The figure shows three views and two pictorial views of one solid part (mm, origin at its lowest corner). Answer the questions. Give positions to 0.01 mm unless a question says otherwise; leave off trailing zeros. Loops run counter-clockwise (first coordinate to the right, second up) from the corner with the lowest first, then second, coordinate; pieces in that order, holes last. Notation, with made-up numbers: (23, -14.75) - (82, -14.75) arc R7 ccw to (82, -9.75) - close; hole circle Ø2 at (34.5, 17.5). An arc over 180 degrees is marked (long way). Write item = value, one per line.
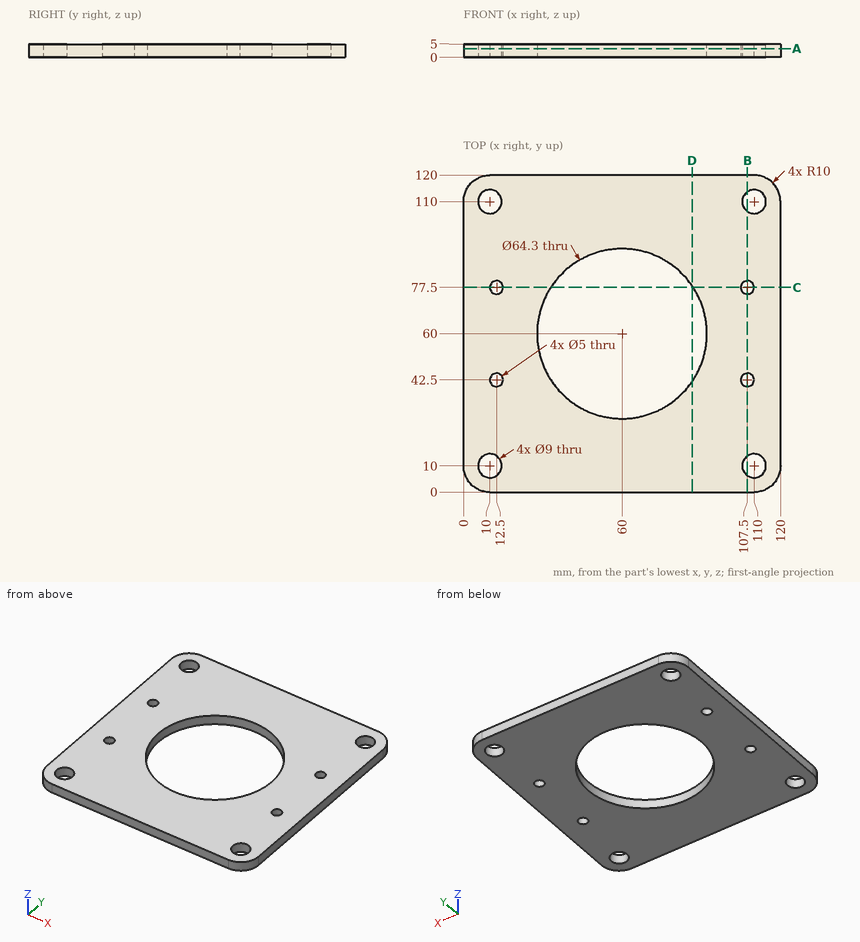
1) Find the intervals of material crossed by probe 1 along X at (y, z) = (6.5, 0.8); probe 2 along Y at (x, z) = (106, 4.4); probe 3 along Y at (x, z) = (74, 0.6), in increasing order.
Output:
probe_1 = 0.63 to 7.17, 12.83 to 107.17, 112.83 to 119.37
probe_2 = 0 to 7.94, 12.06 to 40.5, 44.5 to 75.5, 79.5 to 107.94, 112.06 to 120
probe_3 = 0 to 31.06, 88.94 to 120
2) A cutting plane is placed at C-C on y = 77.5. Determine the outline of the cut face in (x, z), then the cut area to 3 significant figures.
Output:
outline = (0, 0) - (10, 0) - (10, 5) - (0, 5) - close; (15, 0) - (33.03, 0) - (33.03, 5) - (15, 5) - close; (86.97, 0) - (105, 0) - (105, 5) - (86.97, 5) - close; (110, 0) - (120, 0) - (120, 5) - (110, 5) - close
area = 280 mm²
3) A cutting plane is placed at B-B on x = 107.5. Determine the outline of the cut face in (y, z), then the cut area to 3 significant figures.
Output:
outline = (0, 0) - (6.26, 0) - (6.26, 5) - (0, 5) - close; (13.74, 0) - (40, 0) - (40, 5) - (13.74, 5) - close; (45, 0) - (75, 0) - (75, 5) - (45, 5) - close; (80, 0) - (106.26, 0) - (106.26, 5) - (80, 5) - close; (113.74, 0) - (120, 0) - (120, 5) - (113.74, 5) - close
area = 475 mm²
4) A cutting plane is placed at A-A on z = 3.25. Give the number of separate pieces and of enclosed holes in the cut face, then the cut area to 3 significant figures.
Output:
separate_pieces = 1
enclosed_holes = 9
area = 10,700 mm²
5) A cutting plane is placed at D-D on x = 86.5. Determine the outline of the cut face in (y, z), then the cut area to 3 significant figures.
Output:
outline = (0, 0) - (41.8, 0) - (41.8, 5) - (0, 5) - close; (78.2, 0) - (120, 0) - (120, 5) - (78.2, 5) - close
area = 418 mm²
6) This flat-tipped pin is pushed along its axis until it touches: P1, Ø8, axis at x = 10, y = 110, coming from the +Z side. Where does it stop, or does it pass through?
Output:
P1 = through
